```python
from build123d import *

# Parameters (mm, degrees)
SKETCH1_R           = 4.25
BOSS_EXTRUDE1_DEPTH = 2
SKETCH2_R           = 2
BOSS_EXTRUDE2_DEPTH = 6
CUT_EXTRUDE1_DEPTH  = 1
FILLET1_R           = 0.5


with BuildPart() as part:
    # Sketch1 → Boss-Extrude1 (new body)
    with BuildSketch(Plane.XY):
        Circle(SKETCH1_R)
    extrude(amount=-BOSS_EXTRUDE1_DEPTH)

    # Sketch2 → Boss-Extrude2 (add)
    with BuildSketch(Plane(origin=(0, 0, -2), x_dir=(-1, 0, 0), z_dir=(0, 0, -1))):
        with Locations(Location((0, 0, 0), (0, 0, 180))):
            Circle(SKETCH2_R)
    extrude(amount=BOSS_EXTRUDE2_DEPTH)

    # Sketch3 → Cut-Extrude1 (cut)
    with BuildSketch(Plane.XY):
        Polygon((-4.25, -0.25), (-0.25, -0.25), (-0.25, -4.25), (0.125, -4.817995393), (0.25, -4.25), (0.25, -0.25), (4.25, -0.25), (4.809434234, 0), (4.25, 0.25), (0.25, 0.25), (0.25, 4.25), (0, 4.809434234), (-0.25, 4.25), (-0.25, 0.25), (-4.25, 0.25), (-4.9274721, -0.052748768), align=None)
    extrude(amount=-CUT_EXTRUDE1_DEPTH, mode=Mode.SUBTRACT)

    # Fillet1
    fillet1_edges = [part.edges().sort_by_distance(p)[0] for p in [
        (-3.00520382, 3.00520382, 0),
        (-3.00520382, -3.00520382, 0),
        (3.00520382, -3.00520382, 0),
        (3.00520382, 3.00520382, 0),
    ]]
    fillet(fillet1_edges, radius=FILLET1_R)


solid = part.part
```
Here's how the part is built. I have some questions about the finished solid (model axes, mm). A direction names the side the tool comes from. Coordinates: 2 decimals unless noted, no trailing zeros. Loops run counter-clockwise (first coordinate to the right, second up) from the corner with the lowest first, then second, coordinate; pieces in that order, holes last. Notation, with made-up numbers: M -8,64 L 42,64 A31 cw 42,101 Z; hole C 33,30 d9. An arc over 180 degrees is marked long. One line per item, written item: value.
1. Will these pins go through, and if not, where does the flat tip stop? pin 1 Ø0.8 at (x, z) = (2, -0.5) entering from -Y; pin 2 Ø0.5 at (y, z) = (-2, -0.5) entering from -X; pin 3 Ø1.5 at (x, z) = (-1, -6.5) entering from -Y.
Geometry says:
pin 1: stops at y = -3.94
pin 2: stops at x = -3.87
pin 3: stops at y = -1.98
2. On a 3-axis mill with a long thin cutter (end or side, diameter ignored), from which of +Z, -Z, +X, -X, +Y, -Y can I reach the whole of each face in a straight line? I mean faces 1 (the flat face through (-2, 2, 0)), 2 (the flat face through (2.2, -0.25, -0.5)), 3 (the flat face through (2, -1, -2)), 4 (the flat face through (0.25, -2.3, -0.5)), 5 (the flat face through (0, 0, -1)). Say none if no direction works.
Geometry says:
face 1: +Z, +X, -X, +Y, -Y
face 2: +Z, +X, -X
face 3: -Z
face 4: +Z, +Y, -Y
face 5: +Z
3. Please list where these lines run through material, in increasing order: probe 1 along Z at (x, y) = (2.25, -2.25); probe 2 along X at (y, z) = (-2.5, -0.5); probe 3 along X at (y, z) = (-1.5, -1.25).
Geometry says:
probe 1: z = -2 to 0
probe 2: x = -3.44 to -0.25, 0.25 to 3.44
probe 3: x = -3.98 to 3.98
4. Thinking about a two-plate mould opening in Y: for faces 6 (the cylindrical face through (4.054, 1.277, -1.24)), 7 (the flat face through (-2.2, 0.25, -0.5)), 8 (the flat face through (-0.25, 2.3, -0.5)), which applies, +Y half, -Y half, draft (parallel to the pull), parting line (faces both ways), or undercut?
Geometry says:
face 6: parting line
face 7: undercut
face 8: draft
5. Imagine slicing it at C-C (z = -7). List the corners of the cut face in (x, y) for me, and give its area (3 significant figures).
Geometry says:
outline: C 0,0 d4
area: 12.6 mm2
6. Imagine slicing it at A-A (y = 0). List the corners of the cut face in (x, z) for me.
Geometry says:
outline: M -4.25,-2 L -2,-2 L -2,-8 L 2,-8 L 2,-2 L 4.25,-2 L 4.25,-1 L -4.25,-1 Z
